```python
from build123d import *

# Parameters (mm, degrees)
SKETCH1_W           = 20
SKETCH1_H           = 11
SKETCH1_W_2         = 11
SKETCH1_H_2         = 13
BOSS_EXTRUDE1_DEPTH = 15
SKETCH2_R           = 2.5
CUT_EXTRUDE1_DEPTH  = 36
CUT_EXTRUDE2_DEPTH  = 36
CUT_EXTRUDE3_START  = 2
SKETCH1_3_W         = 20
SKETCH1_3_H         = 11
SKETCH1_3_W_2       = 11
SKETCH1_3_H_2       = 13
CUT_EXTRUDE3_DEPTH  = 11
FILLET4_R           = 7
BOSS_EXTRUDE2_REACH = 40.798
SKETCH5_W           = 5
SKETCH5_H           = 2


with BuildPart() as part:
    # Sketch1 → Boss-Extrude1 (new body)
    # profile 1 of 3: a face of its own
    with BuildSketch(Plane.XY):
        Polygon((-12, -15), (-12, 15), (-8, 15), (-8, 0), (8, 0), (8, 15), (12, 15), (12, -15), (7.5, -15), (7.5, -30), (-7.5, -30), (-7.5, -15), align=None)
        with Locations((0, -7.5)):
            Rectangle(SKETCH1_W, SKETCH1_H, mode=Mode.SUBTRACT)
    # profile 2 of 3: a face of its own
    with BuildSketch(Plane.XY):
        with Locations((0, -7.5)):
            Rectangle(SKETCH1_W, SKETCH1_H)
    # profile 3 of 3: a face of its own
    with BuildSketch(Plane.XY):
        with Locations((0, -19.5)):
            Rectangle(SKETCH1_W_2, SKETCH1_H_2)
    extrude(amount=BOSS_EXTRUDE1_DEPTH)

    # Sketch2 → Cut-Extrude1 (cut)
    with BuildSketch(Plane(origin=(12, 0, 0), x_dir=(0, 0, -1), z_dir=(1, 0, 0))):
        with Locations(Location((-7.5, 10, 0), (0, 0, 90))):
            Circle(SKETCH2_R)
        with Locations(Location((-7.5, -25, 0), (0, 0, 180))):
            Circle(SKETCH2_R)
    extrude(amount=-CUT_EXTRUDE1_DEPTH, mode=Mode.SUBTRACT)

    # Sketch3 → Cut-Extrude2 (cut)
    with BuildSketch(Plane(origin=(0, 0, 0), x_dir=(1, 0, 0), z_dir=(0, 1, 0))):
        Polygon((-1.25, 0), (1.25, 0), (1.25, -1.5), (3.5, -1.5), (3.5, -10.5), (-3.5, -10.5), (-3.5, -1.5), (-1.25, -1.5), align=None)
    extrude(amount=-CUT_EXTRUDE2_DEPTH, mode=Mode.SUBTRACT)

    # Sketch1<3> → Cut-Extrude3 (cut)
    with BuildSketch(Plane.XY.offset(CUT_EXTRUDE3_START)):
        with Locations((0, -7.5)):
            Rectangle(SKETCH1_3_W, SKETCH1_3_H)
        with Locations((0, -19.5)):
            Rectangle(SKETCH1_3_W_2, SKETCH1_3_H_2)
    extrude(amount=CUT_EXTRUDE3_DEPTH, mode=Mode.SUBTRACT)

    # Fillet4
    fillet4_edges = [part.edges().sort_by_distance(p)[0] for p in [
        (10, 15, 15),
        (10, 15, 0),
        (-10, 15, 15),
        (-10, 15, 0),
        (4.375, -30, 0),
        (-4.375, -30, 0),
    ]]
    fillet(fillet4_edges, radius=FILLET4_R)

    # Boss-Extrude2: up to this face of the body (flat: up to its plane)
    boss_extrude2_end = Plane(part.part.faces().sort_by_distance((-7.5, -21.9277031, 7.820372358))[0])
    # Sketch5 → Boss-Extrude2 (add, up to the picked face)
    with BuildSketch(Plane(origin=(7.5, 0, 0), x_dir=(0, 0, -1), z_dir=(1, 0, 0)), mode=Mode.PRIVATE) as boss_extrude2_sk1:
        with Locations((-12.5, -31)):
            Rectangle(SKETCH5_W, SKETCH5_H)
    boss_extrude2_tool1 = split(extrude(boss_extrude2_sk1.sketch, amount=-BOSS_EXTRUDE2_REACH, mode=Mode.PRIVATE), bisect_by=boss_extrude2_end, keep=Keep.BOTH, mode=Mode.PRIVATE)
    add(boss_extrude2_tool1.solids().sort_by(Axis((7.5, -31, 12.5), (-1, 0, 0)))[0])


solid = part.part
```
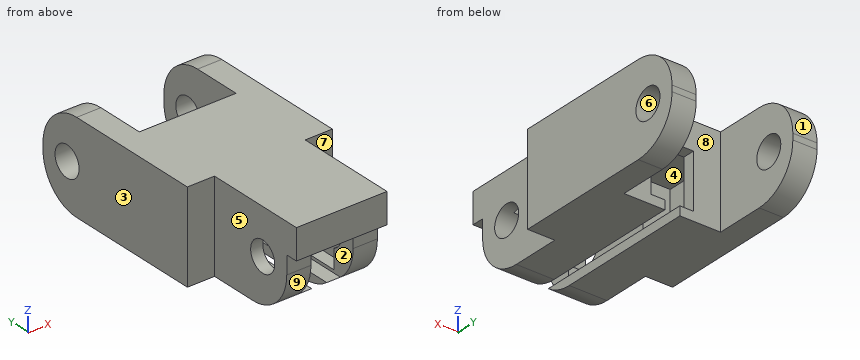
For this review, take the finished solid that the model builds, in its own axes (mm). Face numbers are marked on the shaded views. A direction names the side the tool comes from. Give positions to 0.01 mm unless a question says otherwise; leave off trailing zeros. Write each loop counter-clockwise with the first axis right and the second up, starting at its lowest first coordinate (ties: lowest second). Pieces come first, ordered by that corner, then holes. Notation, with made-up numbers: M 89,69 L 130,69 A12 cw 130,80 Z; hole C 7.25,-4 d5. An arc over 180 degrees is marked long. Answer as a JSON object with one key per item and string values. Group by question number.
Item 1: Tool access review of the marked faces 5, 6, 7, 8 and 9: name each direction out of +Z, -Z, +X, -X, +Y, -Y from which nothing blocks a thin tool from reaching the whole face with its end or side.
Item 2: Consider section A-A on x = 4. Write out the cut boundary in (y, z).
Item 3: For probe 1 along Y at (x, z) = (5.7, 7.5); probe 2 along X at (y, z) = (-5.5, 3.25); probe 3 along X at (y, z) = (-19, 1.75), list the stretches that pass through material, from the lowest coordinate up. Write a range as [from, to].
Item 4: Consider section D-D on z = 4.5. Write out the cut boundary in (x, y).
Item 5: Draft analysis for pull direction X (two halves, no side actions). For the marked faces 1, 2, 3 and 4, state which applies: +X half, -X half, draft (parallel to the pull), parting line (faces both ways), or undercut.
Item 6: For pin 1 Ø9 at (y, z) = (-22.5, 8) entering from -X; pin 2 Ø0.6 at (x, z) = (-0.5, 10.5) entering from +Y; pin 3 Ø2 at (x, z) = (6, 5) entering from -Y; pin 4 Ø4.5 at (y, z) = (10, 7.5) entering from +X, all flat-tipped, find the tip position at first contact; note any pin that passes through.
Item 7: Consider section C-C on y = 10. Write out the cut boundary in (x, z).
Item 8: Consider section B-B on x = -9.25. Write out the cut boundary in (y, z), plus the area to 3 significant figures.
Check result:
{
 "1": {"face 5": "+Z, -Z, -X, -Y", "face 6": "+X, -X", "face 7": "+Z, -Z, +X, -Y", "face 8": "+Z, -Z, +Y", "face 9": "-Z, +X, -X, -Y"},
 "2": {"outline": "M -32,10 L -30,10 L -30,7 A7 ccw -23,0 L 0,0 L 0,15 L -32,15 Z; hole M -26,2 L -2,2 L -2,13 L -26,13 L -26,9.79 A2.5 ccw -26,5.21 Z"},
 "3": {"probe 1": "y = [-30, -27.5], [-22.5, -13], [-2, 0]", "probe 2": "x = [-12, -10], [10, 12]", "probe 3": "x = [-7.5, -3.5], [3.5, 7.5]"},
 "4": {"outline": "M -12,-15 L -7.5,-15 L -7.5,-29.54 L -3.5,-29.54 L -3.5,-26 L -5.5,-26 L -5.5,-13 L -10,-13 L -10,-2 L -3.5,-2 L -3.5,0 L -8,0 L -8,14.54 L -12,14.54 Z; M 3.5,-29.54 L 7.5,-29.54 L 7.5,-15 L 12,-15 L 12,14.54 L 8,14.54 L 8,0 L 3.5,0 L 3.5,-2 L 10,-2 L 10,-13 L 5.5,-13 L 5.5,-26 L 3.5,-26 Z"},
 "5": {"face 1": "draft", "face 2": "undercut", "face 3": "-X half", "face 4": "undercut"},
 "6": {"pin 1": "stops at x = -7.5", "pin 2": "stops at y = 0", "pin 3": "stops at y = -29.93", "pin 4": "passes through"},
 "7": {"outline": "M -12,0.29 L -8,0.29 L -8,5 L -12,5 Z; M -12,10 L -8,10 L -8,14.71 L -12,14.71 Z; M 8,0.29 L 12,0.29 L 12,5 L 8,5 Z; M 8,10 L 12,10 L 12,14.71 L 8,14.71 Z"},
 "8": {"outline": "M -15,0 L 8,0 A7 ccw 15,7 L 15,8 A7 ccw 8,15 L -15,15 Z; hole M -13,2 L -2,2 L -2,13 L -13,13 Z; hole C 10,7.5 d5", "area": "288 mm^2"}
}
